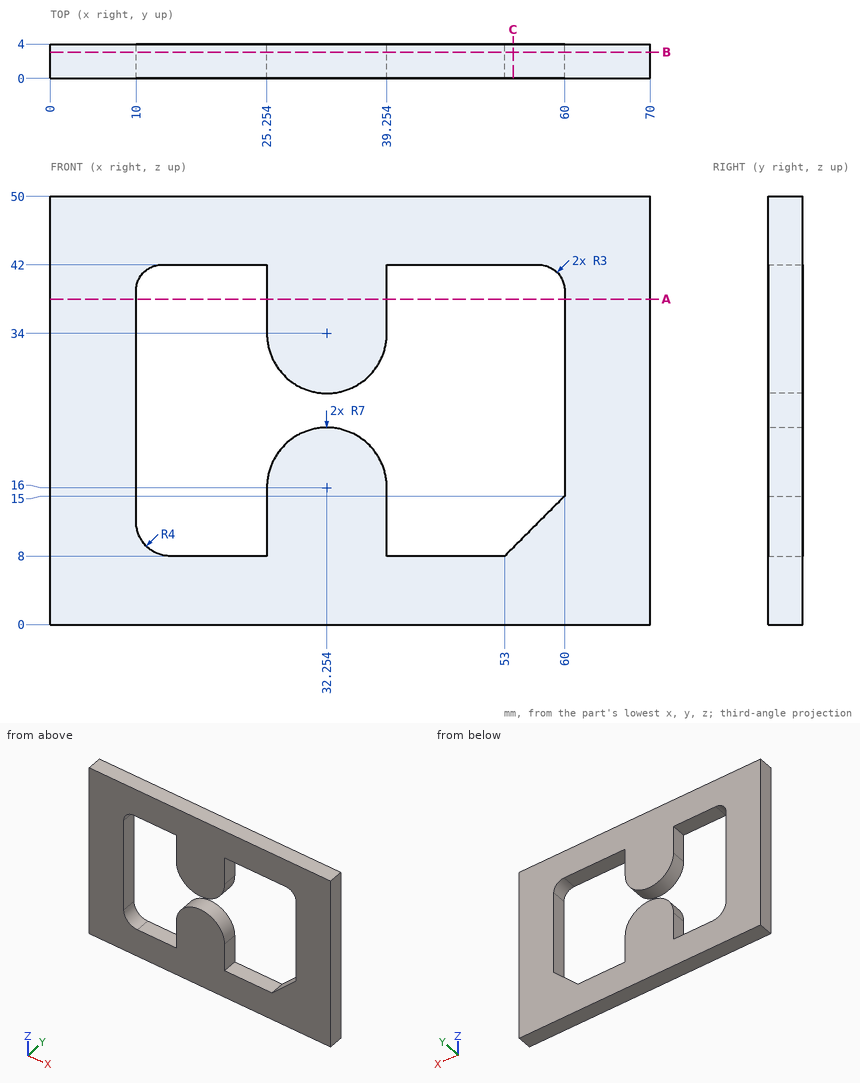
Input: dimensioned drawing with shaded views. Units: mm. Origin: part minimum x, y, z. Coordinates: 2 decimals unless noted, no trailing zeros. Order: outer loops, then holes, each group sorted by start corner. A loop starts at its lowest first (then second) coordinate and runs counter-clockwise, first axis right, second up. Notation, with made-up numbers: (-36.75, 87.5) - (-0.75, 87.5) arc R30 cw to (-0.75, 110.5) - close; hole circle Ø10 at (83, 62.25). An arc over 180 degrees is marked (long way). Put each result on its own line as item: value.
1. Cut plane A-A on z = 38. Return the cut outline in (x, y), then the cut area to 3 significant figures.
Report:
outline: (0, 0) - (10, 0) - (10, 4) - (0, 4) - close; (25.25, 0) - (39.25, 0) - (39.25, 4) - (25.25, 4) - close; (60, 0) - (70, 0) - (70, 4) - (60, 4) - close
area: 136 mm2
2. Cut plane B-B on y = 3.05. Return the cut outline in (x, z).
Report:
outline: (0, 0) - (70, 0) - (70, 50) - (0, 50) - close; hole (10, 12) arc R4 ccw to (14, 8) - (25.25, 8) - (25.25, 16) arc R7 cw to (39.25, 16) - (39.25, 8) - (53, 8) - (60, 15) - (60, 39) arc R3 ccw to (57, 42) - (39.25, 42) - (39.25, 34) arc R7 cw to (25.25, 34) - (25.25, 42) - (13, 42) arc R3 ccw to (10, 39) - close
3. Contact query for a flat-ended pin moving along its axis: pin 1 Ø1.2 at (x, y) = (19.5, 1) entering from -Z. Output: stop coordinate, or through.
Report:
pin 1: stops at z = 0
4. Cut plane C-C on x = 54. Return the cut outline in (y, z), then the cut area to 3 significant figures.
Report:
outline: (0, 0) - (4, 0) - (4, 9) - (0, 9) - close; (0, 42) - (4, 42) - (4, 50) - (0, 50) - close
area: 68.0 mm2
5. Line query: line 1 along X through (y, z) = (0.75, 35); line 2 along Z through (x, y) = (19, 2.2); line 3 along X through (y, z) = (2.05, 30.5). Output: solid intervals per line, ascending.
Report:
line 1: x = 0 to 10, 25.25 to 39.25, 60 to 70
line 2: z = 0 to 8, 42 to 50
line 3: x = 0 to 10, 26.19 to 38.32, 60 to 70
